For this review, take the finished solid that the model builds, in its own axes (mm). Round coordinates to 2 decimals unless told otherwise and drop trailing zeros. Order: outer loops, then holes, each group sorted by start corner. A loop starts at its lowest first (then second) coordinate and runs counter-clockwise, first axis right, second up. Notation, with made-up numbers: M -32,80.25 L 25,80.25 A14 ccw 25,94.25 Z; hole C -30,-0.5 d4. An arc over 180 degrees is marked long. Answer in a Markdown table with one row per item. Add a question column.
```python
from build123d import *

# Parameters (mm, degrees)
F0_W     = 14
F0_H     = 12
F1_DEPTH = 24
F3_DEPTH = 28
F4_DEPTH = 4
F6_DEPTH = 24
F8_DEPTH = 24
F9_R     = 11


with BuildPart() as f1:
    # F0 (on Front) → F1 (new body)
    with BuildSketch(Plane.XZ):
        with Locations((-47.7052051574, 17.2259079414)):
            Rectangle(F0_W, F0_H)
    extrude(amount=F1_DEPTH)

    # F2 (on face) → F3 (join)
    with BuildSketch(Plane.XZ.offset(24)):
        with BuildLine():
            ThreePointArc((-40.7052051574, 11.2764181987), (-40.4564775624, 11.2385675589), (-40.2052051574, 11.2259079414))
            ThreePointArc((-40.2052051574, 11.2259079414), (-38.4374382044, 11.9581409885), (-37.7052051574, 13.7259079414))
            ThreePointArc((-37.7052051574, 13.7259079414), (-38.4374382044, 15.4936748944), (-40.2052051574, 16.2259079414))
            ThreePointArc((-40.2052051574, 16.2259079414), (-40.4564775624, 16.2132483239), (-40.7052051574, 16.1753976842))
            Line((-40.7052051574, 16.1753976842), (-40.7052051574, 11.2764181987))
        make_face()
        with BuildLine():
            ThreePointArc((-40.7052051574, 16.1753976842), (-42.7052051574, 13.7259079414), (-40.7052051574, 11.2764181987))
            Line((-40.7052051574, 11.2764181987), (-40.7052051574, 16.1753976842))
        make_face()
    extrude(amount=-F3_DEPTH)

    # F2 (on face) → F4 (join)
    with BuildSketch(Plane.XZ.offset(24)):
        with BuildLine():
            ThreePointArc((-40.7052051574, 11.2764181987), (-40.4564775624, 11.2385675589), (-40.2052051574, 11.2259079414))
            ThreePointArc((-40.2052051574, 11.2259079414), (-38.4374382044, 11.9581409885), (-37.7052051574, 13.7259079414))
            ThreePointArc((-37.7052051574, 13.7259079414), (-38.4374382044, 15.4936748944), (-40.2052051574, 16.2259079414))
            ThreePointArc((-40.2052051574, 16.2259079414), (-40.4564775624, 16.2132483239), (-40.7052051574, 16.1753976842))
            Line((-40.7052051574, 16.1753976842), (-40.7052051574, 11.2764181987))
        make_face()
        with BuildLine():
            ThreePointArc((-40.7052051574, 16.1753976842), (-42.7052051574, 13.7259079414), (-40.7052051574, 11.2764181987))
            Line((-40.7052051574, 11.2764181987), (-40.7052051574, 16.1753976842))
        make_face()
    extrude(amount=F4_DEPTH)

    # F5 (on face) → F6 (join)
    with BuildSketch(Plane.XZ.offset(24)):
        Polygon((-37.7052051574, 23.2259079414), (-40.7052051574, 23.2259079414), (-40.7052051574, 16.1753976842), (-40.7052051574, 13.2259079414), (-37.7052051574, 13.2259079414), align=None)
    extrude(amount=-F6_DEPTH)

    # F7 (on face) → F8 (join)
    with BuildSketch(Plane.XZ.offset(24)):
        with BuildLine():
            Line((-40.7052051574, 11.2259079414), (-54.7052051574, 11.2259079414))
            Line((-54.7052051574, 11.2259079414), (-54.7052051574, 6.2259079414))
            Line((-54.7052051574, 6.2259079414), (-37.7052051574, 6.2259079414))
            Line((-37.7052051574, 6.2259079414), (-37.7052051574, 13.2259079414))
            Line((-37.7052051574, 13.2259079414), (-37.7557154146, 13.2259079414))
            ThreePointArc((-37.7557154146, 13.2259079414), (-37.7178647749, 13.4746355364), (-37.7052051574, 13.7259079414))
            ThreePointArc((-37.7052051574, 13.7259079414), (-41.7863439875, 15.6623996145), (-40.7052051574, 11.2764181987))
            Line((-40.7052051574, 11.2764181987), (-40.7052051574, 11.2259079414))
        make_face()
    extrude(amount=-F8_DEPTH)

    # F9
    f9_edges = [f1.edges().sort_by_distance(p)[0] for p in [
        (-54.705205, -12, 6.225908),
    ]]
    fillet(f9_edges, radius=F9_R)


solid = f1.part
```
1. To check wall thickness, follow probe 1 along Y at (x, z) = (-47.25, 12.5); probe 2 along Z at (x, y) = (-47, -10); probe 3 along X at (y, z) = (-8, 14.25). State the ranges of each line that lie inside material, in increasing order. Write a range as [from, to].
2. Consider section B-B on z = 12. Write out the cut boundary in (x, y), plus the area to 3 significant figures.
3. Clearance check with flat-ended pins moving along their axes: pin 1 Ø2 at (y, z) = (-13, 9) entering from -X; pin 2 Ø5 at (x, z) = (-49.5, 13) entering from +Y; pin 3 Ø6 at (x, z) = (-49, 13) entering from -Y. State where each tip first meets the part, or that it passes through.
4. The part is to be moulded in two halves that separate along X. For faces 1 (the flat face through (-40, -28, 14)), 2 (the flat face through (-54.705, -12, 20)), 3 (the flat face through (-37.705, -12, 15)), say which applies: pulls with the +X half, pulls with the -X half, needs draft (parallel to the pull), parting line crosses it, or undercut.
5. Consider section C-C on x = -50.5. Write out the cut boundary in (y, z).
6. Consider section D-D on y = -10. Write out the cut boundary in (x, z).
7. Consider section A-A on y = -25.5. Write out the cut boundary in (x, z), plus the area to 3 significant figures.
Solved:
| question | item | result |
|---|---|---|
| 1 | probe 1 | y = [-24, 0] |
| 1 | probe 2 | z = [6.73, 23.23] |
| 1 | probe 3 | x = [-54.3, -37.71] |
| 2 | outline | M -53.38,-24 L -42.01,-24 L -42.01,-28 L -38.4,-28 L -38.4,-24 L -37.71,-24 L -37.71,0 L -38.4,0 L -38.4,4 L -42.01,4 L -42.01,0 L -53.38,0 Z |
| 2 | area | 405 mm^2 |
| 3 | pin 1 | stops at x = -52 |
| 3 | pin 2 | stops at y = 0 |
| 3 | pin 3 | stops at y = -24 |
| 4 | face 1 | needs draft |
| 4 | face 2 | pulls with the -X half |
| 4 | face 3 | pulls with the +X half |
| 5 | outline | M -24,8.58 L 0,8.58 L 0,23.23 L -24,23.23 Z |
| 6 | outline | M -54.71,17.23 A11 ccw -43.71,6.23 L -37.71,6.23 L -37.71,23.23 L -54.71,23.23 Z |
| 7 | outline | C -40.21,13.73 d5 |
| 7 | area | 19.6 mm^2 |
